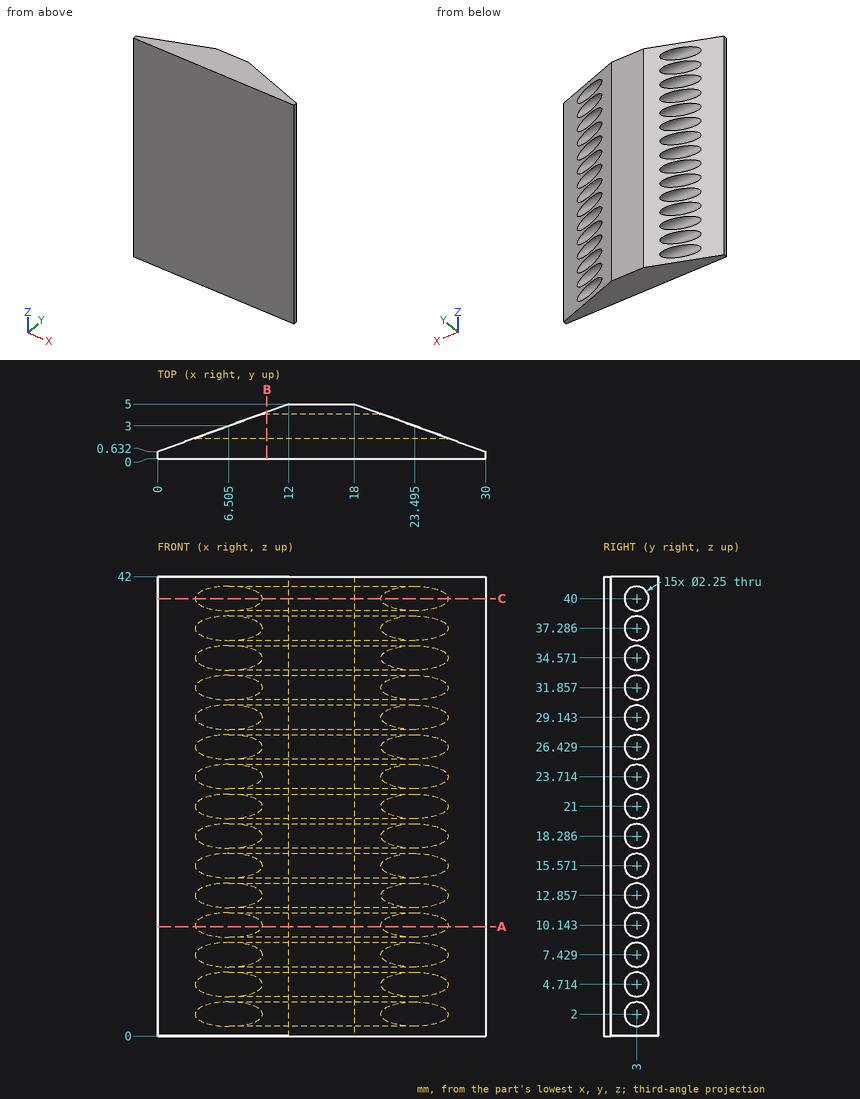
Geometry: see drawing. Coordinates: mm, zero at the bounding-box minimum. Give positions to 0.01 mm unless a question says otherwise; leave off trailing zeros. Write each loop counter-clockwise with the first axis right and the second up, starting at its lowest first coordinate (ties: lowest second). Pieces come first, ordered by that corner, then holes. Notation, with made-up numbers: M 23.5,61.25 L 79.5,61.25 A16 cw 79.5,79.25 Z; hole C 60,14 d8. An arc over 180 degrees is marked long. Answer as a JSON object with one key per item and string values.
Q1. Cut plane B-B, the plane x = 10. Count the separate pieces of the cut face and the enclosed holes in it, then the cut area to 3 significant figures.
Geometry check:
{"separate pieces": "1", "enclosed holes": "15", "area": "120 mm^2"}
Q2. Contact query for a flat-ended pin moving along its axis: P1, Ø5, axis at x = 21.5, z = 12.5, coming from the +Y side. Output: stop coordinate, or through.
Geometry check:
{"P1": "stops at y = 4.64"}
Q3. Ray query, line 1 along Y through (x, z) = (10.5, 21) (1 decimal); line 2 along Y through (x, z) = (17.25, 7); line 3 along Y through (x, z) = (20.75, 11.5). Return the intervals inside material, ascending.
Geometry check:
{"line 1": "y = 0 to 1.9, 4.1 to 4.5", "line 2": "y = 0 to 1.96, 4.04 to 5", "line 3": "y = 0 to 4"}
Q4. Cut plane C-C, the plane z = 40. Return the cut outline in (x, y) (1 decimal).
Geometry check:
{"outline": "M 0,0 L 30,0 L 30,0.6 L 26.6,1.9 L 3.4,1.9 L 0,0.6 Z; M 9.6,4.1 L 20.4,4.1 L 18,5 L 12,5 Z"}
Q5. Cut plane A-A, the plane z = 10. Return the cut outline in (x, y).
Geometry check:
{"outline": "M 0,0 L 30,0 L 30,0.63 L 26.56,1.88 L 3.44,1.88 L 0,0.63 Z; M 9.57,4.12 L 20.43,4.12 L 18,5 L 12,5 Z"}
